from build123d import *

# Parameters (mm, degrees)
SKETCH2_R           = 2.6
BOSS_EXTRUDE1_DEPTH = 5.08
SKETCH3_W           = 100
SKETCH3_H           = 3
BOSS_EXTRUDE2_DEPTH = 10.16


with BuildPart() as part:
    # Sketch2 → Boss-Extrude1 (new body)
    with BuildSketch(Plane.XY):
        with BuildLine():
            Line((-50, -3), (50, -3))
            Line((50, -3), (50, 0))
            Line((50, 0), (8.444744964, 65.520221164))
            ThreePointArc((8.444744964, 65.520221164), (0, 70.1642635), (-8.444744964, 65.520221164))
            Line((-8.444744964, 65.520221164), (-50, 0))
            Line((-50, 0), (-50, -3))
        make_face()
        with Locations((0, 60.1642635)):
            Circle(SKETCH2_R, mode=Mode.SUBTRACT)
        with BuildLine():
            Line((-13.873524959, 51.359417946), (-41.57784754, 7.677978832))
            ThreePointArc((-41.57784754, 7.677978832), (-41.736678897, 2.590632257), (-37.355475058, 0))
            Line((-37.355475058, 0), (-6.5, 0))
            ThreePointArc((-6.5, 0), (-2.964466094, 1.464466094), (-1.5, 5))
            Line((-1.5, 5), (-1.5, 46.645757665))
            ThreePointArc((-1.5, 46.645757665), (-2.267191634, 49.307210903), (-4.333333333, 51.151926277))
            ThreePointArc((-4.333333333, 51.151926277), (-5.426311672, 51.764552693), (-6.434101651, 52.509047243))
            ThreePointArc((-6.434101651, 52.509047243), (-10.41474909, 53.62278713), (-13.873524959, 51.359417946))
        make_face(mode=Mode.SUBTRACT)
        with BuildLine():
            Line((13.873524959, 51.359417946), (41.57784754, 7.677978832))
            ThreePointArc((41.57784754, 7.677978832), (41.736678897, 2.590632257), (37.355475058, 0))
            Line((37.355475058, 0), (6.5, 0))
            ThreePointArc((6.5, 0), (2.964466094, 1.464466094), (1.5, 5))
            Line((1.5, 5), (1.5, 46.645757665))
            ThreePointArc((1.5, 46.645757665), (2.267191634, 49.307210903), (4.333333333, 51.151926277))
            ThreePointArc((4.333333333, 51.151926277), (5.426311672, 51.764552693), (6.434101651, 52.509047243))
            ThreePointArc((6.434101651, 52.509047243), (10.41474909, 53.62278713), (13.873524959, 51.359417946))
        make_face(mode=Mode.SUBTRACT)
    extrude(amount=BOSS_EXTRUDE1_DEPTH)

    # Sketch3 → Boss-Extrude2 (add)
    with BuildSketch(Plane.XY.offset(5.08)):
        with Locations((0, -1.5)):
            Rectangle(SKETCH3_W, SKETCH3_H)
    extrude(amount=BOSS_EXTRUDE2_DEPTH)


solid = part.part
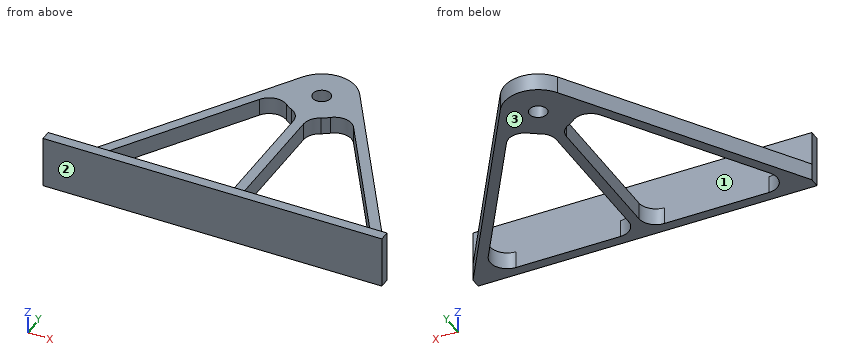
Here's how the part is built. I have some questions about the finished solid (model axes, mm). Face numbers are marked on the shaded views. Coordinates: 2 decimals unless noted, no trailing zeros. Loops run counter-clockwise (first coordinate to the right, second up) from the corner with the lowest first, then second, coordinate; pieces in that order, holes last.
1. Imagine slicing it at D-D, the plane x = 18. Please give me the cut outline in (y, z), and give its area (3 significant figures).
2. If we mould it in two halves opening along Y, with no side actions, what happens to the marked faces 1, 2 and 3? For each: pulls with the +Y half, pulls with the -Y half, needs draft (parallel to the pull), parting line crosses it, or undercut.
3. Imagine slicing it at C-C, the plane z = 2. Please give me the cut outline in (x, y), and give its area (3 significant figures).
4. Imagine slicing it at A-A, the plane x = 0. Please give me the cut outline in (y, z).
5. For P1, Ø1.5, axis at x = 0.5, y = 15.5, coming from the -Z side; P2, Ø1, axis at y = 36.5, z = 6, coming from the -X side; P3, Ø3, axis at x = -34, z = 10, coming from the +Y side; P4, Ø7.5, axis at x = 18.5, z = 5.5, coming from the +Y side, each with a flat end and sliding along its axis, tell me the tip position at first contact or that it passes through.
6. Imagine slicing it at B-B, the plane y = 10.5. Please give me the cut outline in (x, z).
7. I need wall thicknesses on L1, parallel to X at y = 1.5, z = 4; L2, parallel to X at y = 13, z = 4; L3, parallel to Y at x = -31, z = 13.75. Which ranges of each line are inside material? Lowest first, please.
Taken from the geometry:
1. outline: (-3, 0) - (0, 0) - (0, 15.24) - (-3, 15.24) - close; (44.85, 0) - (50.45, 0) - (50.45, 5.08) - (44.85, 5.08) - close
1. area: 74.2 mm2
2. face 1: undercut
2. face 2: pulls with the -Y half
2. face 3: needs draft
3. outline: (-50, -3) - (50, -3) - (50, 0) - (8.44, 65.52) arc R10 ccw to (-8.44, 65.52) - (-50, 0) - close; hole (-41.58, 7.68) arc R5 ccw to (-37.36, 0) - (-6.5, 0) arc R5 ccw to (-1.5, 5) - (-1.5, 46.65) arc R5 ccw to (-4.33, 51.15) arc R10 cw to (-6.43, 52.51) arc R5 ccw to (-13.87, 51.36) - close; hole circle Ø5.2 at (0, 60.16); hole (1.5, 5) arc R5 ccw to (6.5, 0) - (37.36, 0) arc R5 ccw to (41.58, 7.68) - (13.87, 51.36) arc R5 ccw to (6.43, 52.51) arc R10 cw to (4.33, 51.15) arc R5 ccw to (1.5, 46.65) - close
3. area: 1,250 mm2
4. outline: (-3, 0) - (57.56, 0) - (57.56, 5.08) - (0, 5.08) - (0, 15.24) - (-3, 15.24) - close; (62.76, 0) - (70.16, 0) - (70.16, 5.08) - (62.76, 5.08) - close
5. P1: stops at z = 0
5. P2: passes through
5. P3: stops at y = 0
5. P4: stops at y = 55.54
6. outline: (-43.34, 0) - (-39.79, 0) - (-39.79, 5.08) - (-43.34, 5.08) - close; (-1.5, 0) - (1.5, 0) - (1.5, 5.08) - (-1.5, 5.08) - close; (39.79, 0) - (43.34, 0) - (43.34, 5.08) - (39.79, 5.08) - close
7. L1: x = -49.05 to -40.93, -2.93 to 2.93, 40.93 to 49.05
7. L2: x = -41.75 to -38.2, -1.5 to 1.5, 38.2 to 41.75
7. L3: y = -3 to 0
